Part print with two shaded views. Sizes in mm from the minimum x, y, z corner. A direction names the side the tool comes from. Coordinates: 2 decimals unless noted, no trailing zeros. Write each loop counter-clockwise with the first axis right and the second up, starting at its lowest first coordinate (ties: lowest second). Pieces come first, ordered by that corner, then holes. Notation, with made-up numbers: M -15,-14 L 24,-14 A17 cw 24,9 Z; hole C 11,26.5 d1. An arc over 180 degrees is marked long. One line per question, with ' | ' between items. Start each with the question number.
(1) Wall check: probe 1 along Y at (x, z) = (16.5, 4); probe 2 along Z at (x, y) = (7.75, 113) (1 decimal); probe 3 along Z at (x, y) = (17.25, 92) (1 decimal). Give the ranges that are in metal, low to high.
(2) Tool access for the marked faces 1 and 2: list every direction of +Z, -Z, +X, -X, +Y, -Y with a clear straight run to the whole face (end or side of a thin tool).
(3) Cut at A-A (x = 11). Write the cut outline in (y, z).
(4) Flat gauge pins, fed straight in: pin 1 Ø6 at (x, y) = (17.5, 56) entering from -Z (1 decimal); pin 2 Ø1 at (y, z) = (22.5, 4) entering from -X; pin 3 Ø8 at (x, z) = (15, 2) entering from -Y; pin 4 Ø1 at (y, z) = (35.5, 5.5) entering from -X. Where does each tip first touch, or does it go through?
(5) Cut at D-D (x = 2). Write the cut outline in (y, z), plus the area to 3 significant figures.
(6) Cut at B-B (y = 112). Write the cut outline in (x, z).
(7) Cut at C-C (x = 19). Write the cut outline in (y, z).
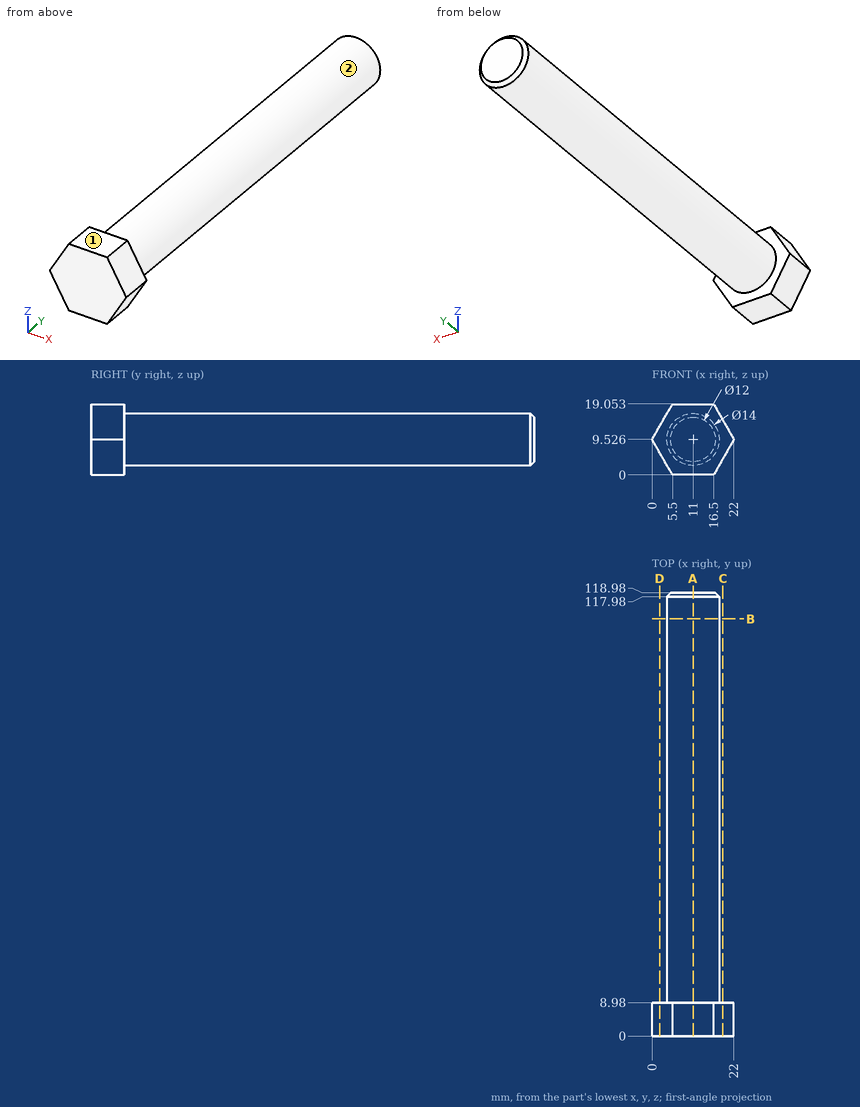
Filled in:
1) probe 1: 0 to 8.98 | probe 2: 3.3 to 15.7 | probe 3: 6.4 to 12.7
2) face 1: +Z, +X, -X, +Y, -Y | face 2: +Y
3) outline: M 0,0 L 8.98,0 L 8.98,2.53 L 117.98,2.53 L 118.98,3.53 L 118.98,15.53 L 117.98,16.53 L 8.98,16.53 L 8.98,19.05 L 0,19.05 Z
4) pin 1: z = 3.5 | pin 2: x = 6.13 | pin 3: y = 0 | pin 4: x = 4.95
5) outline: M 0,6.06 L 8.98,6.06 L 8.98,12.99 L 0,12.99 Z | area: 62.2 mm²
6) outline: C 11,9.53 d14
7) outline: M 0,4.33 L 8.98,4.33 L 8.98,14.72 L 0,14.72 Z
